Read the model definition and answer for the solid it produces. Units are mm, in the model's axes. Face numbers are marked on the shaded views. A direction names the side the tool comes from. Coordinates: 2 decimals unless noted, no trailing zeros. Order: outer loops, then holes, each group sorted by start corner. A loop starts at its lowest first (then second) coordinate and runs counter-clockwise, first axis right, second up.
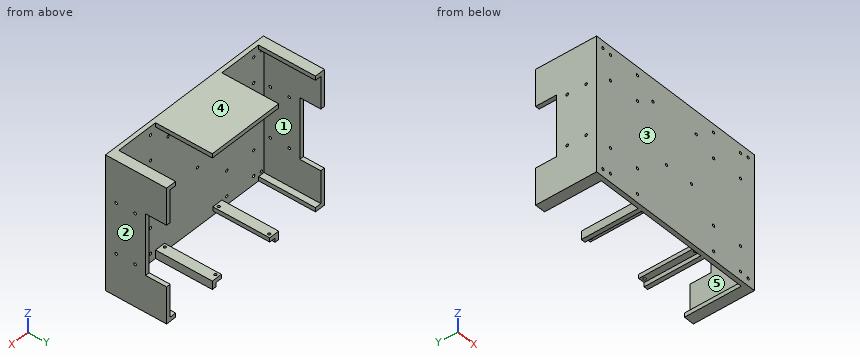
```python
from build123d import *

# Parameters (mm, degrees)
SKETCH_1_W             = 176
SKETCH_1_H             = 128
EXTRUDE_1_DEPTH        = 58
SKETCH_2_W             = 168
SKETCH_2_H             = 120
CUT_EXTRUDE_1_DEPTH    = 54
SKETCH_3_W             = 41
SKETCH_3_H             = 54
CUT_EXTRUDE_2_DEPTH    = 226.219892549
SKETCH_5_W             = 58.134630982
SKETCH_5_H             = 20.010666667
CUT_EXTRUDE_4_DEPTH    = 226.219892549
HOLE_WIZARD_M3_1_D     = 2.5
HOLE_WIZARD_M3_2_D     = 2.5
SKETCH_15_W            = 74
SKETCH_15_H            = 8
EXTRUDE_2_DEPTH        = 54
CUT_EXTRUDE_5_DEPTH    = 54
HOLE_WIZARD_M3_4_D     = 2.5
HOLE_WIZARD_M3_4_DEPTH = 4


with BuildPart() as part:
    # 草图1 → 凸台-拉伸1 (new body)
    with BuildSketch(Plane(origin=(0, 0, 0), x_dir=(1, 0, 0), z_dir=(0, 1, 0))):
        with Locations((88, -64)):
            Rectangle(SKETCH_1_W, SKETCH_1_H)
    extrude(amount=EXTRUDE_1_DEPTH)

    # 草图2 → 切除-拉伸1 (cut)
    with BuildSketch(Plane(origin=(0, 58, 0), x_dir=(1, 0, 0), z_dir=(0, 1, 0))):
        with Locations((88, -64)):
            Rectangle(SKETCH_2_W, SKETCH_2_H)
    extrude(amount=-CUT_EXTRUDE_1_DEPTH, mode=Mode.SUBTRACT)

    # 草图3 → 切除-拉伸2 (cut, through all)
    with BuildSketch(Plane.XY.offset(128)):
        with Locations((30.5, 31)):
            Rectangle(SKETCH_3_W, SKETCH_3_H)
        with Locations((145.5, 31)):
            Rectangle(SKETCH_3_W, SKETCH_3_H)
    extrude(amount=-CUT_EXTRUDE_2_DEPTH, mode=Mode.SUBTRACT)

    # 草图5 → 切除-拉伸4 (cut, through all)
    with BuildSketch(Plane.ZY):
        with Locations((64, 47.994666667)):
            Rectangle(SKETCH_5_W, SKETCH_5_H)
    extrude(amount=-CUT_EXTRUDE_4_DEPTH, mode=Mode.SUBTRACT)

    # M3 螺纹孔1 (through all)
    with Locations(Plane.ZY):
        with Locations((40, 27.989333333), (88, 27.989333333), (88, 10), (40, 10)):
            Hole(HOLE_WIZARD_M3_1_D / 2)

    # M3 螺纹孔2 (through all)
    with Locations(Plane(origin=(0, 4, 0), x_dir=(1, 0, 0), z_dir=(0, 1, 0))):
        with Locations((7, -7), (15.5, -8.05), (15.5, -32.25), (45.5, -32.25), (45.5, -8.05), (15.5, -95.75), (15.5, -119.95), (7, -121), (45.5, -119.95), (45.5, -95.75), (130.5, -119.95), (160.5, -119.95), (160.5, -95.75), (130.5, -95.75), (169, -121), (169, -7), (160.5, -8.05), (160.5, -32.25), (130.5, -32.25), (130.5, -8.05), (105.95, -55.92), (111.03, -106), (62.77, -106), (78.01, -55.92)):
            Hole(HOLE_WIZARD_M3_2_D / 2)

    # 草图15 → 凸台-拉伸2 (add)
    with BuildSketch(Plane(origin=(0, 4, 0), x_dir=(1, 0, 0), z_dir=(0, 1, 0))):
        with Locations((88, -4)):
            Rectangle(SKETCH_15_W, SKETCH_15_H)
    extrude(amount=EXTRUDE_2_DEPTH)

    # 草图16 → 切除-拉伸5 (cut)
    with BuildSketch(Plane(origin=(0, 58, 0), x_dir=(1, 0, 0), z_dir=(0, 1, 0))):
        Polygon((55, 0), (55, -4), (61, -4), (61, -8), (115, -8), (115, -4), (121, -4), (121, 0), align=None)
    extrude(amount=-CUT_EXTRUDE_5_DEPTH, mode=Mode.SUBTRACT)

    # M3 螺纹孔4
    with Locations(Plane(origin=(0, 0, 4), x_dir=(-1, 0, 0), z_dir=(0, 0, -1))):
        with Locations((-118, 55), (-58, 55), (-58, 7), (-118, 7)):
            Hole(HOLE_WIZARD_M3_4_D / 2, depth=HOLE_WIZARD_M3_4_DEPTH)


solid = part.part
```
1) A cutting plane is placed at A-A, the plane y = 18. State how many separate pieces and enclosed holes the cut face has, and give its area (3 significant figures).
A:
separate pieces: 5
enclosed holes: 0
area: 1,530 mm2
2) A cutting plane is placed at B-B, the plane z = 70.5. Determine the outline of the cut face in (x, y).
A:
outline: (0, 0) - (176, 0) - (176, 37.99) - (172, 37.99) - (172, 4) - (4, 4) - (4, 37.99) - (0, 37.99) - close
3) Which of the six approach directions +Z, -Z, +X, -X, +Y, -Y give full straight-line access (tool end or side, diameter ignored) to the marked faces 1 and 2?
A:
face 1: +Y
face 2: +Z, -Z, +X, +Y, -Y
4) Determine the mould class of the marked faces 3, 4 and 5 for opening direction Z: pulls with the +Z half, pulls with the -Z half, needs draft (parallel to the pull), parting line crosses it, or undercut.
A:
face 3: needs draft
face 4: pulls with the +Z half
face 5: undercut
5) Straight lines are drawn through the part: line 1 (Z direction, x = 45.5, y = 0.95); line 2 (Y direction, x = 174, z = 40); line 3 (X direction, y = 55, z = 106). For each, find the intervals that lie inside material, in ascending order.
A:
line 1: z = 0 to 6.8, 9.3 to 31, 33.5 to 94.5, 97 to 118.7, 121.2 to 128
line 2: y = 0 to 8.75, 11.25 to 26.74, 29.24 to 37.99
line 3: x = 0 to 4, 172 to 176
6) A cutting plane is placed at C-C, the plane x = 67.5. Determine the outline of the cut face in (y, z), and give its area (3 significant figures).
A:
outline: (0, 0) - (4, 0) - (4, 124) - (58, 124) - (58, 128) - (0, 128) - close
area: 728 mm2
7) Flat-ended cylindrical pins translate along their axes: pin 1 Ø8 at (x, z) = (46, 47) entering from +Y; pin 2 Ø1 at (x, y) = (122, 34) entering from -Z; pin 3 Ø1.5 at (x, y) = (58, 7) entering from -Z. Find the tip coordinate at first contact, or state that the pin passes through.
A:
pin 1: stops at y = 4
pin 2: stops at z = 0
pin 3: stops at z = 124
